The model under review builds one solid part; all positions refer to its coordinate system, in mm. Face numbers are marked on the shaded views. A direction names the side the tool comes from. Round coordinates to 2 decimals unless told otherwise and drop trailing zeros. Order: outer loops, then holes, each group sorted by start corner. A loop starts at its lowest first (then second) coordinate and runs counter-clockwise, first axis right, second up. Notation, with made-up numbers: (3.25, -16.75) - (52.25, -16.75) arc R13 cw to (52.25, -0.75) - close; hole circle Ø5 at (10, 58.25). An arc over 180 degrees is marked (long way). One line per question, with ' | ' between items. Start each with the question number.
Item 1: Tool access review of the marked faces 3 and 4: name each direction out of +Z, -Z, +X, -X, +Y, -Y from which nothing blocks a thin tool from reaching the whole face with its end or side.
Item 2: Add section A-A on y = 0. State the section outline as (x, z) points.
Item 3: Add section B-B on z = 8. State how many separate pieces and enclosed holes the cut face has, and give its area (3 significant figures).
Item 4: For L1, parallel to Z at x = 0, y = -12.2; L2, parallel to X at y = -20, z = 3; L3, parallel to Y at x = 0, z = 1, list the stretches that pass through material, from the lowest coordinate up. Write a range as [from, to].
Item 5: Draft analysis for pull direction Y (two halves, no side actions). For the marked faces 1 and 2, state which applies: +Y half, -Y half, draft (parallel to the pull), parting line (faces both ways), or undercut.
Item 6: Insertion check: pin 1 Ø6 at (y, z) = (14, 8) entering from -X; pin 2 Ø5 at (x, z) = (-1, 4) entering from +Y; pin 3 Ø3 at (x, z) = (-17.5, 2.5) entering from +Y; pin 4 Ø1 at (y, z) = (9.5, 6.5) entering from -X. Each pin has a flat end and moves straight along its axis. Give the tip position at first contact, or say it passes through.
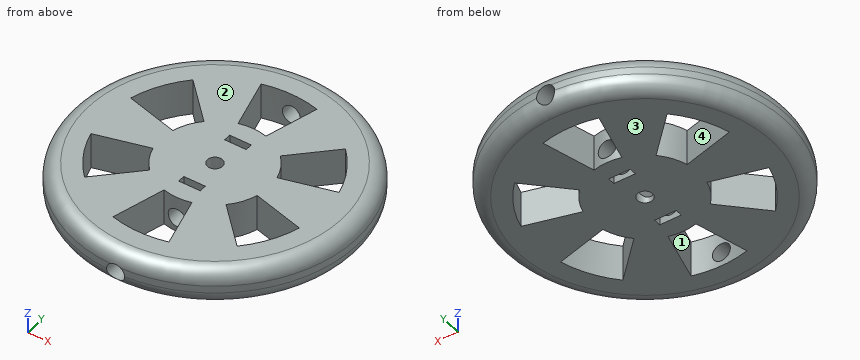
from build123d import *

# Parameters (mm, degrees)
SKETCH1_R               = 39
BOSS_EXTRUDE1_DEPTH     = 10
SKETCH2_R               = 2.1
CUT_EXTRUDE1_DEPTH      = 57.053545829
FILLET1_R               = 4
CUT_EXTRUDE2_DEPTH      = 57.053545829
SKETCH4_W               = 6
SKETCH4_H               = 2
CUT_EXTRUDE3_DEPTH      = 57.053545829
CUT_EXTRUDE4_DEPTH      = 62.886993787
CUT_EXTRUDE4_DEPTH_BACK = 62.886993787
SKETCH5_R               = 2.5


with BuildPart() as part:
    # Sketch1 → Boss-Extrude1 (new body)
    with BuildSketch(Plane.XY):
        Circle(SKETCH1_R)
    extrude(amount=BOSS_EXTRUDE1_DEPTH)

    # Sketch2 → Cut-Extrude1 (cut, through all)
    with BuildSketch(Plane.XY.offset(10)):
        Circle(SKETCH2_R)
    extrude(amount=-CUT_EXTRUDE1_DEPTH, mode=Mode.SUBTRACT)

    # Fillet1
    fillet1_edges = [part.edges().sort_by_distance(p)[0] for p in [
        (-39, 0, 0),
        (-39, 0, 10),
    ]]
    fillet(fillet1_edges, radius=FILLET1_R)

    # Sketch3 → Cut-Extrude2 (cut, through all)
    with BuildSketch(Plane.XY.offset(10)):
        with BuildLine():
            Line((7.764571353, 28.977774789), (3.882285677, 14.488887394))
            ThreePointArc((3.882285677, 14.488887394), (0, 15), (-3.882285677, 14.488887394))
            Line((-3.882285677, 14.488887394), (-7.764571353, 28.977774789))
            ThreePointArc((-7.764571353, 28.977774789), (0, 30), (7.764571353, 28.977774789))
        make_face()
        with BuildLine():
            Line((21.213203436, 21.213203436), (10.606601718, 10.606601718))
            ThreePointArc((10.606601718, 10.606601718), (12.990381057, 7.5), (14.488887394, 3.882285677))
            Line((14.488887394, 3.882285677), (28.977774789, 7.764571353))
            ThreePointArc((28.977774789, 7.764571353), (25.980762114, 15), (21.213203436, 21.213203436))
        make_face()
        with BuildLine():
            Line((28.977774789, -7.764571353), (14.488887394, -3.882285677))
            ThreePointArc((14.488887394, -3.882285677), (12.990381057, -7.5), (10.606601718, -10.606601718))
            Line((10.606601718, -10.606601718), (21.213203436, -21.213203436))
            ThreePointArc((21.213203436, -21.213203436), (25.980762114, -15), (28.977774789, -7.764571353))
        make_face()
        with BuildLine():
            Line((7.764571353, -28.977774789), (3.882285677, -14.488887394))
            ThreePointArc((3.882285677, -14.488887394), (0, -15), (-3.882285677, -14.488887394))
            Line((-3.882285677, -14.488887394), (-7.764571353, -28.977774789))
            ThreePointArc((-7.764571353, -28.977774789), (0, -30), (7.764571353, -28.977774789))
        make_face()
        with BuildLine():
            Line((-21.213203436, -21.213203436), (-10.606601718, -10.606601718))
            ThreePointArc((-10.606601718, -10.606601718), (-12.990381057, -7.5), (-14.488887394, -3.882285677))
            Line((-14.488887394, -3.882285677), (-28.977774789, -7.764571353))
            ThreePointArc((-28.977774789, -7.764571353), (-25.980762114, -15), (-21.213203436, -21.213203436))
        make_face()
        with BuildLine():
            Line((-28.977774789, 7.764571353), (-14.488887394, 3.882285677))
            ThreePointArc((-14.488887394, 3.882285677), (-12.990381057, 7.5), (-10.606601718, 10.606601718))
            Line((-10.606601718, 10.606601718), (-21.213203436, 21.213203436))
            ThreePointArc((-21.213203436, 21.213203436), (-25.980762114, 15), (-28.977774789, 7.764571353))
        make_face()
    extrude(amount=-CUT_EXTRUDE2_DEPTH, mode=Mode.SUBTRACT)

    # Sketch4 → Cut-Extrude3 (cut, through all)
    with BuildSketch(Plane.XY.offset(10)):
        with Locations((0, 9)):
            Rectangle(SKETCH4_W, SKETCH4_H)
        with Locations((0, -9)):
            Rectangle(SKETCH4_W, SKETCH4_H)
    extrude(amount=-CUT_EXTRUDE3_DEPTH, mode=Mode.SUBTRACT)

    # Sketch5 → Cut-Extrude4 (cut, two sides: drawn at the far end of the back side and taken through both)
    with BuildSketch(Plane(origin=(0, 8, 0), x_dir=(1, 0, 0), z_dir=(0, 1, 0)).offset(-CUT_EXTRUDE4_DEPTH_BACK)):
        with Locations(Location((0, -4, 0), (0, 0, 270))):
            Circle(SKETCH5_R)
    extrude(amount=CUT_EXTRUDE4_DEPTH + CUT_EXTRUDE4_DEPTH_BACK, mode=Mode.SUBTRACT)


solid = part.part
Determined:
1) face 3: -Z, +X, -X, +Y, -Y | face 4: +Z, -Z
2) outline: (-39, 4) arc R4 ccw to (-35, 0) - (-2.1, 0) - (-2.1, 2.64) arc R2.5 cw to (-2.1, 5.36) - (-2.1, 10) - (-35, 10) arc R4 ccw to (-39, 6) - close; (2.1, 0) - (35, 0) arc R4 ccw to (39, 4) - (39, 6) arc R4 ccw to (35, 10) - (2.1, 10) - (2.1, 5.36) arc R2.5 cw to (2.1, 2.64) - close
3) separate pieces: 1 | enclosed holes: 9 | area: 3,550 mm2
4) L1: [0, 1.5], [6.5, 10] | L2: [-33.33, -22.36], [-20, -5.36], [5.36, 20], [22.36, 33.33] | L3: [-37.65, -30], [-15, -10], [-8, -2.1], [2.1, 8], [10, 15], [30, 37.65]
5) face 1: undercut | face 2: draft
6) pin 1: x = -37.27 | pin 2: y = 38.98 | pin 3: y = 35.4 | pin 4: x = -37.93
